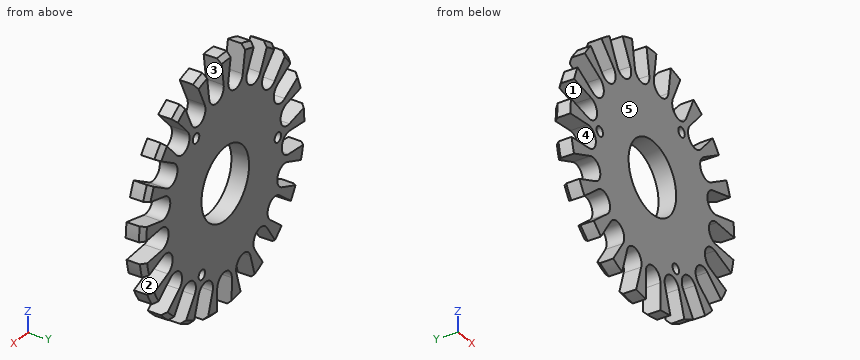
from build123d import *

# Parameters (mm, degrees)
SKETCH1_R            = 28
BOSS_EXTRUDE1_DEPTH  = 4
SKETCH3_R            = 8.125
CUT_EXTRUDE3_DEPTH   = 40.799497484
CUT_EXTRUDE4_DEPTH   = 40.799497484
M2_CLEARANCE_HOLE1_D = 2.2
CHAMFER1_SIZE        = 1


with BuildPart() as part:
    # Sketch1 → Boss-Extrude1 (new body)
    with BuildSketch(Plane(origin=(0, 0, 0), x_dir=(1, 0, 0), z_dir=(0, 1, 0))):
        with Locations(Location((0, 0, 0), (0, 0, 270))):
            Circle(SKETCH1_R)
    extrude(amount=BOSS_EXTRUDE1_DEPTH)

    # Sketch3 → Cut-Extrude3 (cut, through all)
    with BuildSketch(Plane(origin=(0, 0, 0), x_dir=(-1, 0, 0), z_dir=(0, -1, 0))):
        with Locations(Location((0, 0, 0), (0, 0, 90))):
            Circle(SKETCH3_R)
    extrude(amount=-CUT_EXTRUDE3_DEPTH, mode=Mode.SUBTRACT)

    # Sketch4 → Cut-Extrude4 (cut, through all)
    with BuildSketch(Plane(origin=(0, 4, 0), x_dir=(1, 0, 0), z_dir=(0, 1, 0))):
        with BuildLine():
            Line((6.145520364, 27.317257905), (4.3111973, 21.604530107))
            ThreePointArc((4.3111973, 21.604530107), (5.927306058, 18.459717785), (9.07211838, 20.075826543))
            Line((9.07211838, 20.075826543), (10.906441444, 25.788554342))
            ThreePointArc((10.906441444, 25.788554342), (8.560174299, 26.659396392), (6.145520364, 27.317257905))
        make_face()
        with BuildLine():
            Line((-2.179410981, 27.91505271), (-2.248384139, 21.915449164))
            ThreePointArc((-2.248384139, 21.915449164), (0.222875146, 19.386708449), (2.751615861, 21.857967734))
            Line((2.751615861, 21.857967734), (2.820589019, 27.857571279))
            ThreePointArc((2.820589019, 27.857571279), (0.321874739, 27.998149879), (-2.179410981, 27.91505271))
        make_face()
        with BuildLine():
            Line((13.924395256, 24.292204856), (10.48770994, 19.37395374))
            ThreePointArc((10.48770994, 19.37395374), (11.105069816, 15.892500187), (14.586523369, 16.509860063))
            Line((14.586523369, 16.509860063), (18.023208685, 21.428111179))
            ThreePointArc((18.023208685, 21.428111179), (16.037864806, 22.951838542), (13.924395256, 24.292204856))
        make_face()
        with BuildLine():
            Line((20.466026522, 19.108682801), (15.732343527, 15.421916562))
            ThreePointArc((15.732343527, 15.421916562), (15.296099387, 11.913164204), (18.804851745, 11.476920064))
            Line((18.804851745, 11.476920064), (23.53853474, 15.163686303))
            ThreePointArc((23.53853474, 15.163686303), (22.090520644, 17.204909116), (20.466026522, 19.108682801))
        make_face()
        with BuildLine():
            Line((25.189161519, 12.227270422), (19.579089352, 10.099574419))
            ThreePointArc((19.579089352, 10.099574419), (18.128003402, 6.875291302), (21.352286519, 5.424205351))
            Line((21.352286519, 5.424205351), (26.962358687, 7.551901354))
            ThreePointArc((26.962358687, 7.551901354), (26.18033678, 9.929248012), (25.189161519, 12.227270422))
        make_face()
        with BuildLine():
            Line((27.674128974, 4.259411407), (21.686147166, 3.879840768))
            ThreePointArc((21.686147166, 3.879840768), (19.349154761, 1.226518595), (22.002476934, -1.11047381))
            Line((22.002476934, -1.11047381), (27.990458741, -0.730903171))
            ThreePointArc((27.990458741, -0.730903171), (27.943915103, 1.771329648), (27.674128974, 4.259411407))
        make_face()
        with BuildLine():
            Line((27.700128623, -4.086915003), (21.866295637, -2.684633761))
            ThreePointArc((21.866295637, -2.684633761), (18.851048807, -4.531235671), (20.697650716, -7.546482501))
            Line((20.697650716, -7.546482501), (26.531483703, -8.948763742))
            ThreePointArc((26.531483703, -8.948763742), (27.224553939, -6.543979128), (27.700128623, -4.086915003))
        make_face()
        with BuildLine():
            Line((25.264850285, -12.07010108), (20.103527781, -9.0105668))
            ThreePointArc((20.103527781, -9.0105668), (16.67794444, -9.886369762), (17.553747402, -13.311953104))
            Line((17.553747402, -13.311953104), (22.715069906, -16.371487384))
            ThreePointArc((22.715069906, -16.371487384), (24.086171685, -14.277826641), (25.264850285, -12.07010108))
        make_face()
        with BuildLine():
            Line((20.584679125, -18.980805707), (16.554473259, -14.535871436))
            ThreePointArc((16.554473259, -14.535871436), (13.022931519, -14.363056515), (12.850116598, -17.894598255))
            Line((12.850116598, -17.894598255), (16.880322465, -22.339532526))
            ThreePointArc((16.880322465, -22.339532526), (18.807627376, -20.743026599), (20.584679125, -18.980805707))
        make_face()
        with BuildLine():
            Line((14.075468891, -24.204982452), (11.53448114, -18.769600106))
            ThreePointArc((11.53448114, -18.769600106), (8.210773983, -17.563522665), (7.004696543, -20.887229822))
            Line((7.004696543, -20.887229822), (9.545684294, -26.322612168))
            ThreePointArc((9.545684294, -26.322612168), (11.857942838, -25.365117615), (14.075468891, -24.204982452))
        make_face()
        with BuildLine():
            Line((6.315591477, -27.278440283), (5.489599754, -21.335567437))
            ThreePointArc((5.489599754, -21.335567437), (2.669053147, -19.20339275), (0.53687846, -22.023939357))
            Line((0.53687846, -22.023939357), (1.362870183, -27.966812204))
            ThreePointArc((1.362870183, -27.966812204), (3.854628042, -27.733406618), (6.315591477, -27.278440283))
        make_face()
        with BuildLine():
            Line((-2.005453955, -27.928088986), (-1.043056662, -22.005775971))
            ThreePointArc((-1.043056662, -22.005775971), (-3.109824775, -19.136957117), (-5.97864363, -21.20372523))
            Line((-5.97864363, -21.20372523), (-6.941040924, -27.126038245))
            ThreePointArc((-6.941040924, -27.126038245), (-4.491187371, -27.637460737), (-2.005453955, -27.928088986))
        make_face()
        with BuildLine():
            Line((-10.148306003, -26.096204423), (-7.483032915, -20.72067474))
            ThreePointArc((-7.483032915, -20.72067474), (-8.612381119, -17.370118862), (-11.962936997, -18.499467066))
            Line((-11.962936997, -18.499467066), (-14.628210085, -23.874996748))
            ThreePointArc((-14.628210085, -23.874996748), (-12.437941078, -25.085805184), (-10.148306003, -26.096204423))
        make_face()
        with BuildLine():
            Line((-17.389436527, -21.945557575), (-13.258108855, -17.594450627))
            ThreePointArc((-13.258108855, -17.594450627), (-13.349689605, -14.059869319), (-16.884270913, -14.151450068))
            Line((-16.884270913, -14.151450068), (-21.015598585, -18.502557016))
            ThreePointArc((-21.015598585, -18.502557016), (-19.279529136, -20.305165754), (-17.389436527, -21.945557575))
        make_face()
        with BuildLine():
            Line((-23.085439304, -15.844951629), (-17.855143642, -12.904882364))
            ThreePointArc((-17.855143642, -12.904882364), (-16.900819585, -9.500338686), (-20.305363263, -8.54601463))
            Line((-20.305363263, -8.54601463), (-25.535658925, -11.486083895))
            ThreePointArc((-25.535658925, -11.486083895), (-24.408046424, -13.720323238), (-23.085439304, -15.844951629))
        make_face()
        with BuildLine():
            Line((-26.73019949, -8.336452198), (-20.865670559, -7.068658671))
            ThreePointArc((-20.865670559, -7.068658671), (-18.950237578, -4.09666127), (-21.922234979, -2.181228288))
            Line((-21.922234979, -2.181228288), (-27.786763909, -3.449021815))
            ThreePointArc((-27.786763909, -3.449021815), (-27.367801674, -5.916369792), (-26.73019949, -8.336452198))
        make_face()
        with BuildLine():
            Line((-27.999864147, -0.087222404), (-22.02219108, -0.604353634))
            ThreePointArc((-22.02219108, -0.604353634), (-19.3158438, 1.671022478), (-21.591219912, 4.377369759))
            Line((-21.591219912, 4.377369759), (-27.568892979, 4.894500989))
            ThreePointArc((-27.568892979, 4.894500989), (-27.895807644, 2.413279073), (-27.999864147, -0.087222404))
        make_face()
        with BuildLine():
            Line((-26.781618, 8.169757483), (-21.221943281, 5.913650875))
            ThreePointArc((-21.221943281, 5.913650875), (-17.965152534, 7.290228546), (-19.341730205, 10.547019294))
            Line((-19.341730205, 10.547019294), (-24.901404923, 12.803125901))
            ThreePointArc((-24.901404923, 12.803125901), (-25.945148686, 10.528497503), (-26.781618, 8.169757483))
        make_face()
        with BuildLine():
            Line((-23.183707564, 15.700818565), (-18.53603269, 11.906201552))
            ThreePointArc((-18.53603269, 11.906201552), (-15.018178626, 12.261665815), (-15.373642889, 15.779519879))
            Line((-15.373642889, 15.779519879), (-20.021317763, 19.574136892))
            ThreePointArc((-20.021317763, 19.574136892), (-21.689149409, 17.708212725), (-23.183707564, 15.700818565))
        make_face()
        with BuildLine():
            Line((-17.525822971, 21.836793015), (-14.203114251, 16.840833972))
            ThreePointArc((-14.203114251, 16.840833972), (-10.736773642, 16.143600267), (-10.039539937, 19.609940876))
            Line((-10.039539937, 19.609940876), (-13.362248657, 24.605899919))
            ThreePointArc((-13.362248657, 24.605899919), (-15.505974025, 23.314475536), (-17.525822971, 21.836793015))
        make_face()
        with BuildLine():
            Line((-10.310692096, 26.032472578), (-8.608186781, 20.279084389))
            ThreePointArc((-8.608186781, 20.279084389), (-5.501359202, 18.59110499), (-3.813379803, 21.697932569))
            Line((-3.813379803, 21.697932569), (-5.515885118, 27.451320758))
            ThreePointArc((-5.515885118, 27.451320758), (-7.945024803, 26.849144882), (-10.310692096, 26.032472578))
        make_face()
    extrude(amount=-CUT_EXTRUDE4_DEPTH, mode=Mode.SUBTRACT)

    # M2 Clearance Hole1 (through all)
    with Locations(Plane(origin=(0, 0, 0), x_dir=(-1, 0, 0), z_dir=(0, -1, 0))):
        with Locations((-7.995819264, 16.126589047), (17.963945423, -1.138711917), (-9.968126159, -14.98787713)):
            Hole(M2_CLEARANCE_HOLE1_D / 2)

    # Chamfer1
    chamfer1_edges = [part.edges().sort_by_distance(p)[0] for p in [
        (7.945024803, 4, 26.849144882),
        (15.505974025, 4, 23.314475536),
        (21.689149409, 4, 17.708212725),
        (25.945148686, 4, 10.528497503),
        (27.895807644, 4, 2.413279073),
        (27.367801674, 4, -5.916369792),
        (24.408046424, 4, -13.720323238),
        (19.279529136, 4, -20.305165754),
        (12.437941078, 4, -25.085805184),
        (4.491187371, 4, -27.637460737),
        (-3.854628042, 4, -27.733406618),
        (-11.857942838, 4, -25.365117615),
        (-18.807627376, 4, -20.743026599),
        (-24.086171685, 4, -14.277826641),
        (-27.224553939, 4, -6.543979128),
        (-27.943915103, 4, 1.771329648),
        (-26.18033678, 4, 9.929248012),
        (-22.090520644, 4, 17.204909116),
        (-16.037864806, 4, 22.951838542),
        (-8.560174299, 4, 26.659396392),
        (-0.321874739, 4, 27.998149879),
    ]]
    chamfer(chamfer1_edges, length=CHAMFER1_SIZE)


solid = part.part
The model under review builds one solid part; all positions refer to its coordinate system, in mm. Face numbers are marked on the shaded views. A direction names the side the tool comes from. Round coordinates to 2 decimals unless told otherwise and drop trailing zeros. Loops run counter-clockwise (first coordinate to the right, second up) from the corner with the lowest first, then second, coordinate; pieces in that order, holes last. Notation, with made-up numbers: M 71,28.25 L 128,28.25 A22 ccw 128,49.25 Z; hole C 66,50.5 d3. An arc over 180 degrees is marked long. Answer as CSV lines item,"result". Start each with the question number.
Item 1: Wall thickness on line 1 (X direction, y = 0.95, z = 9.5); line 2 (Z direction, x = -7.5, y = 1.7) (3 decimals); line 3 (X direction, y = 1.65, z = 11): over which ranges is each line inside the solid? List them lowest first. Write a range as [from, to].
Item 2: For the marked faces 1, 2 and 3, list the 3-axis set-ups (+Z, -Z, +X, -X, +Y, -Y) from which the entire face can be reached by the end or side of a thin tool; tool diameter is ignored.
Item 3: Insertion check: P1, Ø1.5, axis at y = 1, z = 5.5, coming from the +X side; P2, Ø1, axis at y = 0.5, z = -15.5, coming from the +X side; P3, Ø2.5, axis at x = 8, z = -16.13, coming from the -Y side. Each pin has a flat end and moves straight along its axis. Give the tip position at first contact, or say it passes through.
Item 4: Mouldability with a two-part tool opening along Z and no side actions: class the marked faces 4 and 5 as released by +Z, released by -Z, zero draft, split by the parting line, or undercut.
Item 5: Consider section B-B (z = 10). State how many separate pieces and enclosed holes the cut face has, then the cut area to 3 significant figures.
Item 6: Consider section A-A (z = -1.5). Write out the cut boundary in (x, y), then the cut area to 3 significant figures.
Answer:
1,line 1,"x = [-26.34, -22], [-16.9, 16.96], [20.93, 26.34]"
1,line 2,"z = [-18.846, -3.125], [3.125, 18.466], [20.755, 26.977]"
1,line 3,"x = [-25.75, -24.67], [-16.6, 16.33], [23.46, 25.75]"
2,face 1,"-X, +Y, -Y"
2,face 2,"+X, +Y, -Y"
2,face 3,"+Y, -Y"
3,P1,"stops at x = 19.05"
3,P2,"stops at x = 23.64"
3,P3,"stops at y = 0"
4,face 4,"undercut"
4,face 5,"zero draft"
5,separate pieces,"3"
5,enclosed holes,"0"
5,area,"163 mm^2"
6,outline,"M -19.34,0 L -7.99,0 L -7.99,4 L -19.34,4 Z; M 7.99,0 L 19.35,0 L 19.35,4 L 7.99,4 Z"
6,area,"90.9 mm^2"
